Autodesk Inventor part; units mm, degrees
ref_plane "YZ Plane" through (0, 0, 0) normal (1, 0, 0) x (0, 1, 0)
ref_plane "XZ Plane" through (0, 0, 0) normal (0, 1, 0) x (-1, 0, 0)
ref_plane "XY Plane" through (0, 0, 0) normal (0, 0, 1) x (1, 0, 0)
sketch "Sketch1" plane through (0, 0, 0) normal (0, 0, 1) x (1, 0, 0)
  circle A0 centre (-5.8379, -1.3582) radius 2
  circle A1 centre (54.1621, -1.3582) radius 2
  line L0 (81.6621, 21.6418) -> (111.6621, 21.6418)
  line L1 (111.6621, 21.6418) -> (111.6621, 26.6418)
  line L2 (81.6621, 26.6418) -> (111.6621, 26.6418)
  line L3 (81.6621, 21.6418) -> (81.6621, 26.6418)
  line L4 (-3.3379, 21.6418) -> (51.6621, 21.6418)
  line L5 (51.6621, 21.6418) -> (51.6621, 26.6418)
  line L6 (-3.3379, 26.6418) -> (51.6621, 26.6418)
  line L7 (-3.3379, 21.6418) -> (-3.3379, 26.6418)
  line L8 (-86.3379, 21.6418) -> (-33.3379, 21.6418)
  line L9 (-33.3379, 21.6418) -> (-33.3379, 26.6418)
  line L10 (-86.3379, 26.6418) -> (-33.3379, 26.6418)
  line L11 (-86.3379, 21.6418) -> (-86.3379, 26.6418)
  line L12 (-171.3379, 21.6418) -> (-116.3379, 21.6418)
  line L13 (-116.3379, 21.6418) -> (-116.3379, 26.6418)
  line L14 (-171.3379, 26.6418) -> (-116.3379, 26.6418)
  line L15 (-171.3379, 21.6418) -> (-171.3379, 26.6418)
  line L16 (-231.3379, 21.6418) -> (-201.3379, 21.6418)
  line L17 (-201.3379, 21.6418) -> (-201.3379, 26.6418)
  line L18 (-231.3379, 26.6418) -> (-201.3379, 26.6418)
  line L19 (-231.3379, 21.6418) -> (-231.3379, 26.6418)
  line L20 (126.1621, -31.3589) -> (-245.8379, -31.3589)
  line L21 (-247.8379, -29.3589) -> (-247.8379, 34.6418)
  line L22 (128.1621, -29.3589) -> (128.1621, 34.6418)
  line L23 (-247.8379, 34.6418) -> (128.1621, 34.6418)
  arc A2 (-247.8379, -29.3589) -> (-245.8379, -31.3589) centre (-245.8379, -29.3589) ccw
  arc A3 (126.1621, -31.3589) -> (128.1621, -29.3589) centre (126.1621, -29.3589) ccw
  line L24 (123.1621, -23.3589) -> (123.1621, -8.3597)
  line L25 (123.1621, -8.3597) -> (118.1621, -8.3597)
  line L26 (118.1621, -23.3589) -> (118.1621, -8.3597)
  line L27 (123.1621, -23.3589) -> (118.1621, -23.3589)
  line L28 (123.1621, 11.6403) -> (123.1621, 26.6418)
  line L29 (123.1621, 26.6418) -> (118.1621, 26.6418)
  line L30 (118.1621, 11.6403) -> (118.1621, 26.6418)
  line L31 (123.1621, 11.6403) -> (118.1621, 11.6403)
  line L32 (-237.8379, -23.3589) -> (-237.8379, -8.3597)
  line L33 (-237.8379, -8.3597) -> (-242.8379, -8.3597)
  line L34 (-242.8379, -23.3589) -> (-242.8379, -8.3597)
  line L35 (-237.8379, -23.3589) -> (-242.8379, -23.3589)
  line L36 (-237.8379, 11.6403) -> (-237.8379, 26.6418)
  line L37 (-237.8379, 26.6418) -> (-242.8379, 26.6418)
  line L38 (-242.8379, 11.6403) -> (-242.8379, 26.6418)
  line L39 (-237.8379, 11.6403) -> (-242.8379, 11.6403)
  line L40 (-201.8409, 14.8575) -> (-185.8409, 14.8575)
  line L41 (-185.8409, 19.8575) -> (-201.8409, 19.8575)
  line L42 (-85.8409, 14.8575) -> (-101.8409, 14.8575)
  line L43 (-101.8409, 19.8575) -> (-85.8409, 19.8575)
  line L44 (-176.8409, 14.8575) -> (-110.8409, 14.8575)
  line L45 (-110.8409, 19.8575) -> (-176.8409, 19.8575)
  arc A4 (-178.8409, 16.8575) -> (-176.8409, 14.8575) centre (-176.8409, 16.8575) ccw
  arc A5 (-108.8409, 17.8575) -> (-110.8409, 19.8575) centre (-110.8409, 17.8575) ccw
  arc A6 (-110.8409, 14.8575) -> (-108.8409, 16.8575) centre (-110.8409, 16.8575) ccw
  arc A7 (-103.8409, 16.8575) -> (-101.8409, 14.8575) centre (-101.8409, 16.8575) ccw
  arc A8 (-101.8409, 19.8575) -> (-103.8409, 17.8575) centre (-101.8409, 17.8575) ccw
  arc A9 (-83.8409, 17.8575) -> (-85.8409, 19.8575) centre (-85.8409, 17.8575) ccw
  arc A10 (-85.8409, 14.8575) -> (-83.8409, 16.8575) centre (-85.8409, 16.8575) ccw
  arc A11 (-183.8409, 17.8575) -> (-185.8409, 19.8575) centre (-185.8409, 17.8575) ccw
  arc A12 (-185.8409, 14.8575) -> (-183.8409, 16.8575) centre (-185.8409, 16.8575) ccw
  arc A13 (-203.8409, 16.8575) -> (-201.8409, 14.8575) centre (-201.8409, 16.8575) ccw
  arc A14 (-201.8409, 19.8575) -> (-203.8409, 17.8575) centre (-201.8409, 17.8575) ccw
  arc A15 (-176.8409, 19.8575) -> (-178.8409, 17.8575) centre (-176.8409, 17.8575) ccw
  line L46 (-203.8409, 16.8575) -> (-183.8409, 16.8575)
  line L47 (-183.8409, 17.8575) -> (-203.8409, 17.8575)
  line L48 (-178.8409, 16.8575) -> (-108.8409, 16.8575)
  line L49 (-108.8409, 17.8575) -> (-178.8409, 17.8575)
  line L50 (-103.8409, 16.8575) -> (-83.8409, 16.8575)
  line L51 (-83.8409, 17.8575) -> (-103.8409, 17.8575)
  line L52 (57.1591, 19.8575) -> (-8.8409, 19.8575)
  line L53 (-8.8409, 14.8575) -> (57.1591, 14.8575)
  line L54 (59.1591, 17.8575) -> (-10.8409, 17.8575)
  line L55 (-10.8409, 16.8575) -> (59.1591, 16.8575)
  arc A16 (59.1591, 17.8575) -> (57.1591, 19.8575) centre (57.1591, 17.8575) ccw
  arc A17 (57.1591, 14.8575) -> (59.1591, 16.8575) centre (57.1591, 16.8575) ccw
  arc A18 (64.1591, 16.8575) -> (66.1591, 14.8575) centre (66.1591, 16.8575) ccw
  arc A19 (66.1591, 19.8575) -> (64.1591, 17.8575) centre (66.1591, 17.8575) ccw
  line L56 (82.1591, 14.8575) -> (66.1591, 14.8575)
  line L57 (66.1591, 19.8575) -> (82.1591, 19.8575)
  arc A20 (82.1591, 14.8575) -> (84.1591, 16.8575) centre (82.1591, 16.8575) ccw
  arc A21 (84.1591, 17.8575) -> (82.1591, 19.8575) centre (82.1591, 17.8575) ccw
  line L58 (-33.8409, 14.8575) -> (-17.8409, 14.8575)
  line L59 (-17.8409, 19.8575) -> (-33.8409, 19.8575)
  arc A22 (-10.8409, 16.8575) -> (-8.8409, 14.8575) centre (-8.8409, 16.8575) ccw
  arc A23 (-8.8409, 19.8575) -> (-10.8409, 17.8575) centre (-8.8409, 17.8575) ccw
  arc A24 (-17.8409, 14.8575) -> (-15.8409, 16.8575) centre (-17.8409, 16.8575) ccw
  arc A25 (-15.8409, 17.8575) -> (-17.8409, 19.8575) centre (-17.8409, 17.8575) ccw
  arc A26 (-33.8409, 19.8575) -> (-35.8409, 17.8575) centre (-33.8409, 17.8575) ccw
  line L60 (-35.8409, 16.8575) -> (-15.8409, 16.8575)
  line L61 (-15.8409, 17.8575) -> (-35.8409, 17.8575)
  arc A27 (-35.8409, 16.8575) -> (-33.8409, 14.8575) centre (-33.8409, 16.8575) ccw
  line L62 (64.1591, 16.8575) -> (84.1591, 16.8575)
  line L63 (84.1591, 17.8575) -> (64.1591, 17.8575)
  circle A28 centre (-173.8379, -1.3582) radius 2
  circle A29 centre (-113.8379, -1.3582) radius 2
  line L64 (-237.8379, -31.3589) -> (-242.8379, -31.3589)
  point P0 (24.1621, -1.3582)
  point P1 (-203.8409, 14.8575)
  point P2 (-203.8409, 19.8575)
  point P3 (-35.8409, 14.8575)
  point P4 (-35.8409, 19.8575)
  point P5 (-143.8379, -1.3582)
  dimension "d36" = 4
  dimension "d37" = 4
  dimension "d40" = 30
  dimension "d41" = 30
  dimension "d48" = 2
  dimension "d53" = 2
  dimension "d55" = 8
  dimension "d56" = 5
  dimension "d57" = 2
  dimension "d58" = 5
  dimension "d59" = 2
  dimension "d60" = 376
  dimension "d63" = 28
  dimension "d64" = 28
  dimension "d65" = 28
  dimension "d66" = 4
  dimension "d67" = 4
  dimension "d68" = 30
  dimension "d69" = 30
  dimension "d70" = 74
  dimension "d71" = 74
  dimension "d72" = 28
  dimension "d73" = 28
  dimension "d74" = 2.5
  dimension "d75" = 2.5
  dimension "d76" = 2.5
  dimension "d77" = 0
extrude "Extrusion1" add sketch "Sketch1" along normal blind 5
properties part number "case bottom front" material "Nylon, molybdenum disulphide"
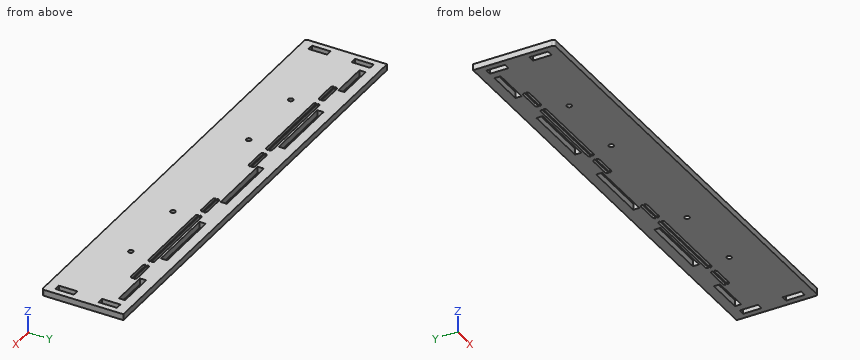
The model under review builds one solid part; all positions refer to its coordinate system, in mm. Give positions to 0.01 mm unless a question says otherwise; leave off trailing zeros. Loops run counter-clockwise (first coordinate to the right, second up) from the corner with the lowest first, then second, coordinate; pieces in that order, holes last. Notation, with made-up numbers: (72.5, 19.25) -> (83.5, 19.25) arc R20 cw to (83.5, 36.25) -> close; hole circle Ø3 at (-33, -1.75). An arc over 180 degrees is marked (long way). Put each result on its own line as item: value. Start each with the question number.
1. Clearance check with flat-ended pins moving along their axes: P1, Ø3, axis at x = -100.5, y = -7, coming from the -Z side; P2, Ø3.5, axis at x = -173.84, y = -1.36, coming from the +Z side. State where each tip first meets the part, or that it passes through.
2. Wall thickness on probe 1 along Y at (x, z) = (-145, 3); probe 2 along X at (y, z) = (-12.5, 1.6); probe 3 along Y at (x, z) = (-190.5, 2.5): over which ranges is each line inside the solid? List them lowest first.
3. We need section B-B on y = -15. State the section outline as (x, z) points.
4. We need section A-A on x = -124.5. State the section outline as (y, z) points.
5. We need section C-C on x = -24.5. State the section outline as (y, z) points, then the cut area to 3 significant figures.
6. We need section D-D on x = -80.5. State the section outline as (y, z) points.
Determined:
1. P1: z = 0
1. P2: through
2. probe 1: -31.36 to 14.86, 16.86 to 17.86, 19.86 to 21.64, 26.64 to 34.64
2. probe 2: -247.84 to -242.84, -237.84 to 118.16, 123.16 to 128.16
2. probe 3: -31.36 to 14.86, 16.86 to 17.86, 19.86 to 34.64
3. outline: (-247.84, 0) -> (-242.84, 0) -> (-242.84, 5) -> (-247.84, 5) -> close; (-237.84, 0) -> (118.16, 0) -> (118.16, 5) -> (-237.84, 5) -> close; (123.16, 0) -> (128.16, 0) -> (128.16, 5) -> (123.16, 5) -> close
4. outline: (-31.36, 0) -> (14.86, 0) -> (14.86, 5) -> (-31.36, 5) -> close; (16.86, 0) -> (17.86, 0) -> (17.86, 5) -> (16.86, 5) -> close; (19.86, 0) -> (21.64, 0) -> (21.64, 5) -> (19.86, 5) -> close; (26.64, 0) -> (34.64, 0) -> (34.64, 5) -> (26.64, 5) -> close
5. outline: (-31.36, 0) -> (14.86, 0) -> (14.86, 5) -> (-31.36, 5) -> close; (16.86, 0) -> (17.86, 0) -> (17.86, 5) -> (16.86, 5) -> close; (19.86, 0) -> (34.64, 0) -> (34.64, 5) -> (19.86, 5) -> close
5. area: 310 mm^2
6. outline: (-31.36, 0) -> (21.64, 0) -> (21.64, 5) -> (-31.36, 5) -> close; (26.64, 0) -> (34.64, 0) -> (34.64, 5) -> (26.64, 5) -> close
